from build123d import *

# Parameters (mm, degrees)
SKETCH1_R               = 40
BOSS_EXTRUDE1_DEPTH     = 50
SKETCH4_R               = 3
CUT_EXTRUDE2_DEPTH      = 15
CIRPATTERN1_COUNT       = 8
SKETCH5_R               = 2.5
CUT_EXTRUDE5_DEPTH      = 15
SKETCH6_R               = 37.5
CUT_EXTRUDE6_DEPTH      = 35
CUT_EXTRUDE9_REACH      = 104.47
CUT_EXTRUDE9_END_RADIUS = 37.5
SKETCH7_R               = 3
CIRPATTERN3_COUNT       = 6


with BuildPart() as part:
    # Sketch1 → Boss-Extrude1 (new, symmetric)
    with BuildSketch(Plane(origin=(0, 0, 0), x_dir=(0, 0, -1), z_dir=(1, 0, 0))):
        Circle(SKETCH1_R)
    extrude(amount=BOSS_EXTRUDE1_DEPTH, both=True)

    # Sketch4 → Cut-Extrude2 (cut)
    with BuildSketch(Plane(origin=(0, 40, 0), x_dir=(1, 0, 0), z_dir=(0, 1, 0))):
        with Locations(Location((0, 0, 0), (0, 0, 270))):
            Circle(SKETCH4_R)
    cut_extrude2 = extrude(amount=-CUT_EXTRUDE2_DEPTH, mode=Mode.SUBTRACT)

    # CirPattern1: Cut-Extrude2 ×8 about axis
    cirpattern1_axis = Axis((0, 0, 0), (1, 0, 0))
    for i in range(1, CIRPATTERN1_COUNT):
        add(cut_extrude2.rotate(cirpattern1_axis, i * 360 / CIRPATTERN1_COUNT), mode=Mode.SUBTRACT)

    # Sketch5 → Cut-Extrude5 (cut)
    with BuildSketch(Plane.ZY.offset(50)):
        with Locations((14.852428205, 26.06540574)):
            Circle(SKETCH5_R)
        with Locations((29.999517634, 0.170122737)):
            Circle(SKETCH5_R)
        with Locations((15.147089429, -25.895283004)):
            Circle(SKETCH5_R)
        with Locations((-14.852428205, -26.06540574)):
            Circle(SKETCH5_R)
        with Locations((-29.999517634, -0.170122737)):
            Circle(SKETCH5_R)
        with Locations((-15.147089429, 25.895283004)):
            Circle(SKETCH5_R)
    extrude(amount=-CUT_EXTRUDE5_DEPTH, mode=Mode.SUBTRACT)

    # Sketch6 → Cut-Extrude6 (cut)
    with BuildSketch(Plane(origin=(50, 0, 0), x_dir=(0, 0, -1), z_dir=(1, 0, 0))):
        Circle(SKETCH6_R)
    extrude(amount=-CUT_EXTRUDE6_DEPTH, mode=Mode.SUBTRACT)

    # Cut-Extrude9: up to this cylinder (the profile starts outside it)
    cut_extrude9_end = Plane(origin=(30, 0, 0), z_dir=(1, 0, 0)) * Cylinder(CUT_EXTRUDE9_END_RADIUS, 284.94, mode=Mode.PRIVATE)
    # Sketch7 → Cut-Extrude9 (cut, up to the surface)
    with BuildSketch(Plane(origin=(0, 40, 0), x_dir=(1, 0, 0), z_dir=(0, 1, 0)), mode=Mode.PRIVATE) as cut_extrude9_sk1:
        with Locations(Location((30, 0, 0), (0, 0, 270))):
            Circle(SKETCH7_R)
    cut_extrude9_tool1 = extrude(cut_extrude9_sk1.sketch, amount=-CUT_EXTRUDE9_REACH, mode=Mode.PRIVATE) - cut_extrude9_end
    cut_extrude9 = cut_extrude9_tool1.solids().sort_by_distance((30, 40, 0))[0]
    add(cut_extrude9, mode=Mode.SUBTRACT)

    # CirPattern3: Cut-Extrude9 ×6 about axis
    cirpattern3_axis = Axis((50, 0, 0), (-1, 0, 0))
    for i in range(1, CIRPATTERN3_COUNT):
        add(cut_extrude9.rotate(cirpattern3_axis, i * 360 / CIRPATTERN3_COUNT), mode=Mode.SUBTRACT)


solid = part.part
Work out the finished part from the listing and answer in its coordinate system (mm). A direction names the side the tool comes from. Coordinates: 2 decimals unless noted, no trailing zeros. Order: outer loops, then holes, each group sorted by start corner. A loop starts at its lowest first (then second) coordinate and runs counter-clockwise, first axis right, second up. Notation, with made-up numbers: (73, -1.75) - (126, -1.75) arc R28 ccw to (126, 36.25) - close; hole circle Ø3 at (2.5, 69). An arc over 180 degrees is marked (long way). Put each result on its own line as item: value. Start each with the question number.
1) Find section C-C (y = 33). Give the vertices of the cut face in (x, z), plus the area to 3 significant figures.
2) Flat-ended cylindrical pins translate along their axes: pin 1 (8 mm diameter, centred on y = 29, z = -6, fed in from +X); pin 2 (6 mm diameter, centred on x = -4, z = -20, fed in from -Y); pin 3 (3 mm diameter, centred on x = -0.5, y = -1, fed in from -Z). Find the tip coordinate at first contact, or state that the pin passes through.
3) Find the intervals of material crossed by line 1 (X direction, y = 39.1, z = 0); line 2 (Y direction, x = -37, z = -13); line 3 (X direction, y = -14, z = 28.5), in increasing order. Write a range as from..to.
4) Find section B-B (x = 30). Give the vertices of the cut face in (y, z), plus the area to 3 significant figures.
5) Find section D-D (x = -41). Give the vertices of the cut face in (y, z).
6) Find section A-A (z = 0). Give the vertices of the cut face in (x, y), plus the area to 4 significant figures.
7) For a pull along Y with two mould halves and no side action, classify faces 1 (the flat face through (50, 36, -12)), 2 (the cylindrical face through (30.9, 21.83, -32.09)), 3 (the flat face through (0, -25, 0)) as released by +Y, released by -Y, zero draft, split by the parting line, or undercut.
8) For faces 4 (the cylindrical face through (-42.6, 24.37, -17.13)), 5 (the flat face through (15, 1, 1)), 6 (the cylindrical face through (-1.8, -2.4, -32.6)), 7 (the cylindrical face through (0.9, -32.61, -2.86)), determine the directions among +Z, -Z, +X, -X, +Y, -Y from which every point of the face is accessible in a straight line to the end or side of a thin tool.
Results list:
1. outline: (-50, -22.61) - (50, -22.61) - (50, -17.81) - (15, -17.81) - (15, 17.81) - (50, 17.81) - (50, 22.61) - (-50, 22.61) - close; hole circle Ø6 at (0, 0)
1. area: 3,250 mm^2
2. pin 1: stops at x = 15
2. pin 2: stops at y = -36.21
2. pin 3: stops at z = -25
3. line 1: x = -50..-3, 3..27, 33..50
3. line 2: y = -37.83..-27.74, -24.39..24.61, 27.18..37.83
3. line 3: x = -50..15
4. outline: (-39.89, -3) arc R40 ccw to (-22.54, -33.04) - (-21.29, -30.87) arc R37.5 cw to (-37.38, -3) - close; (-39.89, 3) - (-37.38, 3) arc R37.5 cw to (-21.29, 30.87) - (-22.54, 33.04) arc R40 ccw to start; (-17.35, -36.04) arc R40 ccw to (17.35, -36.04) - (16.09, -33.87) arc R37.5 cw to (-16.09, -33.87) - close; (-17.35, 36.04) - (-16.09, 33.87) arc R37.5 cw to (16.09, 33.87) - (17.35, 36.04) arc R40 ccw to start; (21.29, -30.87) - (22.54, -33.04) arc R40 ccw to (39.89, -3) - (37.38, -3) arc R37.5 cw to start; (21.29, 30.87) arc R37.5 cw to (37.38, 3) - (39.89, 3) arc R40 ccw to (22.54, 33.04) - close
4. area: 519 mm^2
5. outline: circle Ø80 at (0, 0); hole circle Ø5 at (-26.07, -14.85); hole circle Ø5 at (-25.9, 15.15); hole circle Ø5 at (-0.17, -30); hole circle Ø5 at (0.17, 30); hole circle Ø5 at (25.9, -15.15); hole circle Ø5 at (26.07, 14.85)
6. outline: (-50, -40) - (-3, -40) - (-3, -25) - (3, -25) - (3, -40) - (27, -40) - (27, -37.5) - (15, -37.5) - (15, 37.5) - (27, 37.5) - (27, 40) - (3, 40) - (3, 25) - (-3, 25) - (-3, 40) - (-50, 40) - close; (33, -40) - (50, -40) - (50, -37.5) - (33, -37.5) - close; (33, 37.5) - (50, 37.5) - (50, 40) - (33, 40) - close
6. area: 5,165 mm^2
7. face 1: zero draft
7. face 2: undercut
7. face 3: released by -Y
8. face 4: -X
8. face 5: +X
8. face 6: -Z
8. face 7: -Y
